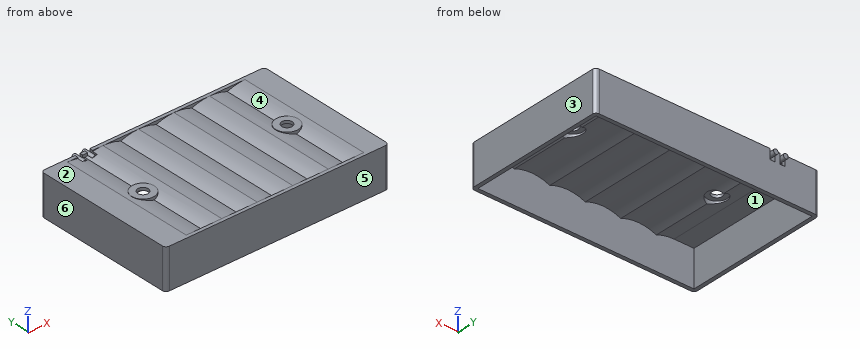
```python
from build123d import *

# Parameters (mm, degrees)
EXTRUDE_1_DEPTH                = 54.7
SKETCH_2_W                     = 1.5
SKETCH_2_H                     = 1.473886678
EXTRUDE_2_DEPTH                = 7.15
SKETCH_3_W                     = 0.15
SKETCH_3_H                     = 1.473886678
EXTRUDE_3_DEPTH                = 7.15
SKETCH_4_W                     = 7.15
SKETCH_4_H                     = 56.35
EXTRUDE_4_DEPTH                = 1.5
SKETCH_5_W                     = 2.973886678
SKETCH_5_H                     = 56.35
EXTRUDE_5_DEPTH                = 14.3
CUT_EXTRUDE_1_DEPTH            = 54.7
SKETCH_7_W                     = 2.973886678
SKETCH_7_H                     = 56.35
EXTRUDE_6_DEPTH                = 14.3
CUT_EXTRUDE_2_DEPTH            = 54.7
SKETCH_9_W                     = 2.973886678
SKETCH_9_H                     = 56.35
EXTRUDE_7_DEPTH                = 14.3
CUT_EXTRUDE_3_DEPTH            = 54.7
SKETCH_11_W                    = 2.973886678
SKETCH_11_H                    = 56.35
EXTRUDE_8_DEPTH                = 14.3
CUT_EXTRUDE_4_DEPTH            = 54.7
EXTRUDE_9_DEPTH                = 7.15
CUT_EXTRUDE_5_DEPTH            = 54.7
CUT_EXTRUDE_6_DEPTH            = 55
CUT_EXTRUDE_7_DEPTH            = 55
CUT_EXTRUDE_8_DEPTH            = 55
CUT_EXTRUDE_9_DEPTH            = 55
CUT_EXTRUDE_10_DEPTH           = 55
SKETCH_20_W                    = 71.5
SKETCH_20_H                    = 1.5
EXTRUDE_10_DEPTH               = 13.126113322
SKETCH_21_W                    = 71.5
SKETCH_21_H                    = 0.15
EXTRUDE_11_DEPTH               = 13.126113322
SKETCH_22_W                    = 16.1
SKETCH_22_H                    = 56.35
EXTRUDE_12_DEPTH               = 9.5
SKETCH_23_W                    = 16.1
SKETCH_23_H                    = 56.35
EXTRUDE_13_DEPTH               = 9
SKETCH_24_W                    = 14.6
SKETCH_24_H                    = 54.7
CUT_EXTRUDE_11_DEPTH           = 8
SKETCH_25_W                    = 14.6
SKETCH_25_H                    = 54.7
CUT_EXTRUDE_12_DEPTH           = 7.5
SKETCH_26_W                    = 90
SKETCH_26_H                    = 16.1
EXTRUDE_14_DEPTH               = 1.35
SKETCH_27_W                    = 4.58
SKETCH_27_H                    = 1.352189545
SKETCH_28_W                    = 4.58
SKETCH_28_H                    = 1.352189545
HOLE_WIZARD_M3_5_1_D           = 4.2
HOLE_WIZARD_M3_5_1_CBORE_D     = 8
HOLE_WIZARD_M3_5_1_CBORE_DEPTH = 1.873886678
FILLET_1_R                     = 1.5
SKETCH_32_W                    = 2
SKETCH_32_H                    = 4
CUT_EXTRUDE_13_DEPTH           = 3.5
SKETCH_35_R                    = 0.95
EXTRUDE_15_DEPTH               = 5


with BuildPart() as part:
    # 草图1 → 凸台-拉伸1 (new body)
    with BuildSketch(Plane(origin=(0, 27.35, 0), x_dir=(1, 0, 0), z_dir=(0, 1, 0))):
        with BuildLine():
            Line((28.85, -5.076113322), (28.85, -6.55))
            Line((28.85, -6.55), (36, -6.55))
            ThreePointArc((36, -6.55), (32.349834184, -6.177694996), (28.85, -5.076113322))
        make_face()
    extrude(amount=-EXTRUDE_1_DEPTH)

    # 草图2 → 凸台-拉伸2 (add)
    with BuildSketch(Plane(origin=(28.85, 0, 0), x_dir=(0, -1, 0), z_dir=(-1, 0, 0))):
        with Locations((28.1, 5.813056661)):
            Rectangle(SKETCH_2_W, SKETCH_2_H)
    extrude(amount=-EXTRUDE_2_DEPTH)

    # 草图3 → 凸台-拉伸3 (add)
    with BuildSketch(Plane(origin=(28.85, 0, 0), x_dir=(0, -1, 0), z_dir=(-1, 0, 0))):
        with Locations((-27.425, 5.813056661)):
            Rectangle(SKETCH_3_W, SKETCH_3_H)
    extrude(amount=-EXTRUDE_3_DEPTH)

    # 草图4 → 凸台-拉伸4 (add)
    with BuildSketch(Plane.XY.offset(6.55)):
        with Locations((32.425, -0.675)):
            Rectangle(SKETCH_4_W, SKETCH_4_H)
    extrude(amount=EXTRUDE_4_DEPTH)

    # 草图5 → 凸台-拉伸5 (add)
    with BuildSketch(Plane.ZY.offset(-28.85)):
        with Locations((6.563056661, -0.675)):
            Rectangle(SKETCH_5_W, SKETCH_5_H)
    extrude(amount=EXTRUDE_5_DEPTH)

    # 草图6 → 切除-拉伸1 (cut)
    with BuildSketch(Plane.XZ.offset(27.35)):
        with BuildLine():
            Line((14.55, 5.076113322), (28.85, 5.076113322))
            ThreePointArc((28.85, 5.076113322), (21.7, 6.55), (14.55, 5.076113322))
        make_face()
    extrude(amount=-CUT_EXTRUDE_1_DEPTH, mode=Mode.SUBTRACT)

    # 草图7 → 凸台-拉伸6 (add)
    with BuildSketch(Plane.ZY.offset(-14.55)):
        with Locations((6.563056661, -0.675)):
            Rectangle(SKETCH_7_W, SKETCH_7_H)
    extrude(amount=EXTRUDE_6_DEPTH)

    # 草图8 → 切除-拉伸2 (cut)
    with BuildSketch(Plane.XZ.offset(27.35)):
        with BuildLine():
            Line((0.25, 5.076113322), (14.55, 5.076113322))
            ThreePointArc((14.55, 5.076113322), (7.4, 6.55), (0.25, 5.076113322))
        make_face()
    extrude(amount=-CUT_EXTRUDE_2_DEPTH, mode=Mode.SUBTRACT)

    # 草图9 → 凸台-拉伸7 (add)
    with BuildSketch(Plane.ZY.offset(-0.25)):
        with Locations((6.563056661, -0.675)):
            Rectangle(SKETCH_9_W, SKETCH_9_H)
    extrude(amount=EXTRUDE_7_DEPTH)

    # 草图10 → 切除-拉伸3 (cut)
    with BuildSketch(Plane.XZ.offset(27.35)):
        with BuildLine():
            Line((-14.05, 5.076113322), (0.25, 5.076113322))
            ThreePointArc((0.25, 5.076113322), (-6.9, 6.55), (-14.05, 5.076113322))
        make_face()
    extrude(amount=-CUT_EXTRUDE_3_DEPTH, mode=Mode.SUBTRACT)

    # 草图11 → 凸台-拉伸8 (add)
    with BuildSketch(Plane.ZY.offset(14.05)):
        with Locations((6.563056661, -0.675)):
            Rectangle(SKETCH_11_W, SKETCH_11_H)
    extrude(amount=EXTRUDE_8_DEPTH)

    # 草图12 → 切除-拉伸4 (cut)
    with BuildSketch(Plane.XZ.offset(27.35)):
        with BuildLine():
            Line((-28.35, 5.076113322), (-14.05, 5.076113322))
            ThreePointArc((-14.05, 5.076113322), (-21.2, 6.55), (-28.35, 5.076113322))
        make_face()
    extrude(amount=-CUT_EXTRUDE_4_DEPTH, mode=Mode.SUBTRACT)

    # 草图13 → 凸台-拉伸9 (add)
    with BuildSketch(Plane.ZY.offset(28.35)):
        with BuildLine():
            Line((5.076113322, 27.35), (5.076113322, 27.5))
            Line((5.076113322, 27.5), (8.05, 27.5))
            Line((8.05, 27.5), (8.05, -28.85))
            Line((8.05, -28.85), (5.076113322, -28.85))
            Line((5.076113322, -28.85), (5.076113322, -27.35))
            add(Edge.make_bspline(
                [(5.076113322, -27.35), (5.076113322, -9.116666667), (5.076113322, 9.116666667), (5.076113322, 27.35)],
                knots=[0, 0, 0, 0, 1, 1, 1, 1], degree=3))
        make_face()
    extrude(amount=EXTRUDE_9_DEPTH)

    # 草图14 → 切除-拉伸5 (cut)
    with BuildSketch(Plane.XZ.offset(27.35)):
        with BuildLine():
            Line((-35.5, 5.076113322), (-28.35, 5.076113322))
            ThreePointArc((-28.35, 5.076113322), (-31.849834184, 6.177694996), (-35.5, 6.55))
            Line((-35.5, 6.55), (-35.5, 5.076113322))
        make_face()
    extrude(amount=-CUT_EXTRUDE_5_DEPTH, mode=Mode.SUBTRACT)

    # 草图15 → 切除-拉伸6 (cut)
    with BuildSketch(Plane(origin=(0, 27.5, 0), x_dir=(-1, 0, 0), z_dir=(0, 1, 0))):
        with BuildLine():
            Line((21.2, 8.05), (6.9, 8.05))
            ThreePointArc((6.9, 8.05), (10.538369022, 7.708982887), (14.05, 6.697810455))
            ThreePointArc((14.05, 6.697810455), (17.561630978, 7.708982887), (21.2, 8.05))
        make_face()
    extrude(amount=-CUT_EXTRUDE_6_DEPTH, mode=Mode.SUBTRACT)

    # 草图16 → 切除-拉伸7 (cut)
    with BuildSketch(Plane(origin=(0, 27.5, 0), x_dir=(-1, 0, 0), z_dir=(0, 1, 0))):
        with BuildLine():
            Line((6.9, 8.05), (-7.4, 8.05))
            ThreePointArc((-7.4, 8.05), (-3.761630978, 7.708982887), (-0.25, 6.697810455))
            ThreePointArc((-0.25, 6.697810455), (3.261630978, 7.708982887), (6.9, 8.05))
        make_face()
    extrude(amount=-CUT_EXTRUDE_7_DEPTH, mode=Mode.SUBTRACT)

    # 草图17 → 切除-拉伸8 (cut)
    with BuildSketch(Plane(origin=(0, 27.5, 0), x_dir=(-1, 0, 0), z_dir=(0, 1, 0))):
        with BuildLine():
            Line((-7.4, 8.05), (-21.7, 8.05))
            ThreePointArc((-21.7, 8.05), (-18.061630978, 7.708982887), (-14.55, 6.697810455))
            ThreePointArc((-14.55, 6.697810455), (-11.038369022, 7.708982887), (-7.4, 8.05))
        make_face()
    extrude(amount=-CUT_EXTRUDE_8_DEPTH, mode=Mode.SUBTRACT)

    # 草图18 → 切除-拉伸9 (cut)
    with BuildSketch(Plane(origin=(0, 27.5, 0), x_dir=(-1, 0, 0), z_dir=(0, 1, 0))):
        with BuildLine():
            Line((-21.7, 8.05), (-36, 8.05))
            ThreePointArc((-36, 8.05), (-32.361630978, 7.708982887), (-28.85, 6.697810455))
            ThreePointArc((-28.85, 6.697810455), (-25.338369022, 7.708982887), (-21.7, 8.05))
        make_face()
    extrude(amount=-CUT_EXTRUDE_9_DEPTH, mode=Mode.SUBTRACT)

    # 草图19 → 切除-拉伸10 (cut)
    with BuildSketch(Plane(origin=(0, 27.5, 0), x_dir=(-1, 0, 0), z_dir=(0, 1, 0))):
        with BuildLine():
            Line((35.5, 8.05), (21.2, 8.05))
            ThreePointArc((21.2, 8.05), (24.838369022, 7.708982887), (28.35, 6.697810455))
            ThreePointArc((28.35, 6.697810455), (31.861630978, 7.708982887), (35.5, 8.05))
        make_face()
    extrude(amount=-CUT_EXTRUDE_10_DEPTH, mode=Mode.SUBTRACT)

    # 草图20 → 凸台-拉伸10 (add)
    with BuildSketch(Plane(origin=(0, 0, 5.076113322), x_dir=(-1, 0, 0), z_dir=(0, 0, -1))):
        with Locations((-0.25, -28.1)):
            Rectangle(SKETCH_20_W, SKETCH_20_H)
    extrude(amount=EXTRUDE_10_DEPTH)

    # 草图21 → 凸台-拉伸11 (add)
    with BuildSketch(Plane(origin=(0, 0, 5.076113322), x_dir=(-1, 0, 0), z_dir=(0, 0, -1))):
        with Locations((-0.25, 27.425)):
            Rectangle(SKETCH_21_W, SKETCH_21_H)
    extrude(amount=EXTRUDE_11_DEPTH)

    # 草图22 → 凸台-拉伸12 (add)
    with BuildSketch(Plane.ZY.offset(35.5)):
        with Locations((0, -0.675)):
            Rectangle(SKETCH_22_W, SKETCH_22_H)
    extrude(amount=EXTRUDE_12_DEPTH)

    # 草图23 → 凸台-拉伸13 (add)
    with BuildSketch(Plane(origin=(36, 0, 0), x_dir=(0, 0, -1), z_dir=(1, 0, 0))):
        with Locations((0, -0.675)):
            Rectangle(SKETCH_23_W, SKETCH_23_H)
    extrude(amount=EXTRUDE_13_DEPTH)

    # 草图24 → 切除-拉伸11 (cut)
    with BuildSketch(Plane(origin=(-35.5, 0, 0), x_dir=(0, 0, -1), z_dir=(1, 0, 0))):
        with Locations((0.75, 0)):
            Rectangle(SKETCH_24_W, SKETCH_24_H)
    extrude(amount=-CUT_EXTRUDE_11_DEPTH, mode=Mode.SUBTRACT)

    # 草图25 → 切除-拉伸12 (cut)
    with BuildSketch(Plane.ZY.offset(-36)):
        with Locations((-0.75, 0)):
            Rectangle(SKETCH_25_W, SKETCH_25_H)
    extrude(amount=-CUT_EXTRUDE_12_DEPTH, mode=Mode.SUBTRACT)

    # 草图26 → 凸台-拉伸14 (add)
    with BuildSketch(Plane(origin=(0, 27.5, 0), x_dir=(-1, 0, 0), z_dir=(0, 1, 0))):
        Rectangle(SKETCH_26_W, SKETCH_26_H)
    extrude(amount=EXTRUDE_14_DEPTH)

    # 草图27 → 旋转1 (revolve)
    with BuildSketch(Plane(origin=(0, 0, 0), x_dir=(1, 0, 0), z_dir=(0, 1, 0))):
        with Locations((-31.29, -7.373905228)):
            Rectangle(SKETCH_27_W, SKETCH_27_H)
    revolve(axis=Axis((-29, 0, 8.05), (0, 0, -1)))

    # 草图28 → 旋转2 (revolve)
    with BuildSketch(Plane(origin=(0, 0, 0), x_dir=(1, 0, 0), z_dir=(0, 1, 0))):
        with Locations((31.29, -7.373905228)):
            Rectangle(SKETCH_28_W, SKETCH_28_H)
    revolve(axis=Axis((29, 0, 6.697810455), (0, 0, 1)))

    # M3.5 六角头机械螺钉的柱形沉头孔1 (through all)
    with Locations(Plane(origin=(0, 0, 5.076113322), x_dir=(-1, 0, 0), z_dir=(0, 0, -1))):
        with Locations((-29, 0), (29, 0)):
            CounterBoreHole(HOLE_WIZARD_M3_5_1_D / 2, HOLE_WIZARD_M3_5_1_CBORE_D / 2, HOLE_WIZARD_M3_5_1_CBORE_DEPTH)

    # 圆角1
    fillet_1_edges = [part.edges().sort_by_distance(p)[0] for p in [
        (-45, -28.85, 0),
        (45, -28.85, 0),
        (45, 28.85, 0),
        (-45, 28.85, 0),
    ]]
    fillet(fillet_1_edges, radius=FILLET_1_R)

    # 草图32 → 切除-拉伸13 (cut)
    with BuildSketch(Plane(origin=(0, 28.85, 0), x_dir=(1, 0, 0), z_dir=(0, 1, 0))):
        with Locations((-30.35, -6.05)):
            Rectangle(SKETCH_32_W, SKETCH_32_H)
        with Locations((-26.35, -6.05)):
            Rectangle(SKETCH_32_W, SKETCH_32_H)
    extrude(amount=-CUT_EXTRUDE_13_DEPTH, mode=Mode.SUBTRACT)

    # 草图35 → 凸台-拉伸15 (add)
    with BuildSketch(Plane(origin=(0, 25.35, 0), x_dir=(1, 0, 0), z_dir=(0, 1, 0))):
        with Locations(Location((-30.35, -6.641832766, 0), (0, 0, 74.804666508))):
            Circle(SKETCH_35_R)
        with Locations(Location((-26.35, -6.641832766, 0), (0, 0, 105.195333492))):
            Circle(SKETCH_35_R)
    extrude(amount=EXTRUDE_15_DEPTH)


solid = part.part
```
CAD build for the part. Positions are in the model's coordinates, mm. Face numbers are marked on the shaded views. A direction names the side the tool comes from. Round coordinates to 2 decimals unless told otherwise and drop trailing zeros. Loops run counter-clockwise (first coordinate to the right, second up) from the corner with the lowest first, then second, coordinate; pieces in that order, holes last. Notation, with made-up numbers: (-19.5, 78.25) - (16.5, 78.25) arc R16 ccw to (16.5, 100.25) - close; hole circle Ø9 at (-21.5, 12.25). An arc over 180 degrees is marked (long way). Return JSON: item names as keys, results as strings. Group by question number.
Q1. Tool access for the marked faces 1 and 2: list every direction of +Z, -Z, +X, -X, +Y, -Y with a clear straight run to the whole face (end or side of a thin tool).
Q2. Drill centre lines: line 1 along Y through (x, z) = (-29, 7.35); line 2 along Y through (x, z) = (-41, -6.25); line 3 along X through (y, z) = (26, 3.25). Where is each one in solid material? Low to high. Write a range as [from, to].
Q3. Two-plate mould, pull along X, no slides. Class the marked faces 3, 4, 5 and 6: +X half, -X half, draft (parallel to the pull), parting line (faces both ways), or undercut.
Q4. Band-saw the part on A-A on z = -3.75. Give the cut face in (x, y), plus the area to 3 significant figures.
Q5. Band-saw the part on B-B on y = 6. Give the cut face in (x, z).
Q6. Flat gauge pins, fed straight in: pin 1 Ø6.5 at (x, y) = (-38.5, 7.5) entering from -Z; pin 2 Ø5 at (x, y) = (-4, 16) entering from -Z; pin 3 Ø1.5 at (x, y) = (-17.5, 4) entering from -Z. Where does each tip first touch, or does it go through?
Q7. Band-saw the part on D-D on y = 0. Give the number of separate pieces and of enclosed holes in the cut face, plus the area to 3 significant figures.
Q8. Band-saw the part on C-C on x = -2.5. Give the cut face in (y, z).
Solutions:
{
 "1": {"face 1": "-Z", "face 2": "+Z, +X, -X, +Y, -Y"},
 "2": {"line 1": "y = [-28.85, -27.5], [-4.58, -2.1], [2.1, 4.58], [27.5, 28.85]", "line 2": "y = [-28.85, -27.35], [27.35, 28.85]", "line 3": "x = [-45, -43.5], [43.5, 45]"},
 "3": {"face 3": "+X half", "face 4": "undercut", "face 5": "draft", "face 6": "-X half"},
 "4": {"outline": "(-45, -27.35) arc R1.5 ccw to (-43.5, -28.85) - (43.5, -28.85) arc R1.5 ccw to (45, -27.35) - (45, 27.35) arc R1.5 ccw to (43.5, 28.85) - (-43.5, 28.85) arc R1.5 ccw to (-45, 27.35) - close; hole (-43.5, -27.35) - (43.5, -27.35) - (43.5, 27.35) - (-43.5, 27.35) - close", "area": "432 mm^2"},
 "5": {"outline": "(-45, -8.05) - (-43.5, -8.05) - (-43.5, 6.55) - (-35.5, 6.55) arc R18.08 cw to (-28.35, 5.08) arc R18.08 cw to (-14.05, 5.08) arc R18.08 cw to (0.25, 5.08) arc R18.08 cw to (14.55, 5.08) arc R18.08 cw to (28.85, 5.08) arc R18.08 cw to (36, 6.55) - (43.5, 6.55) - (43.5, -8.05) - (45, -8.05) - (45, 8.05) - (36, 8.05) arc R19.58 ccw to (28.85, 6.7) arc R19.58 ccw to (14.55, 6.7) arc R19.58 ccw to (0.25, 6.7) arc R19.58 ccw to (-14.05, 6.7) arc R19.58 ccw to (-28.35, 6.7) arc R19.58 ccw to (-35.5, 8.05) - (-45, 8.05) - close"},
 "6": {"pin 1": "stops at z = 6.55", "pin 2": "stops at z = 5.72", "pin 3": "stops at z = 5.99"},
 "7": {"separate pieces": "3", "enclosed holes": "0", "area": "165 mm^2"},
 "8": {"outline": "(-28.85, -8.05) - (-27.35, -8.05) - (-27.35, 6.01) - (27.35, 6.01) - (27.35, -8.05) - (28.85, -8.05) - (28.85, 8.05) - (27.5, 8.05) - (27.5, 7.55) - (-27.5, 7.55) - (-27.5, 8.05) - (-28.85, 8.05) - close"}
}
